Geometry: final body of the model. Coordinates: model frame, mm. A direction names the side the tool comes from. Give positions to 0.01 mm unless a question says otherwise; leave off trailing zeros. Write each loop counter-clockwise with the first axis right and the second up, starting at its lowest first coordinate (ties: lowest second). Pieces come first, ordered by that corner, then holes. Notation, with made-up numbers: (-30.75, -5.5) -> (-12.75, -5.5) arc R23 ccw to (-12.75, 13.5) -> close; hole circle Ø11 at (10, 25). An arc over 180 degrees is marked (long way). Answer as a JSON object with one key per item and string values. Group by question number.
(1) Contact query for flat-ended pins moving along their axis: pin 1 Ø6 at (x, y) = (8.5, 68) entering from +Z; pin 2 Ø7 at (x, z) = (-36.25, -33.1) entering from +Y. Output: stop coordinate, or through.
(2) Set-up query: faces 1 (the face through (44.424, 47.566, -5.07)), 2 (the face through (-0.79, 7.4, -35.99)), 3 (the face through (-39.2, 109.93, -30.39)). Return all of +Z, -Z, +X, -X, +Y, -Y with unobstructed straight access to the full face (end or side cutting, diameter ignored); none if empty.
(3) Section query A-A on y = 10. Output: boundary loops of the cut face in (x, z).
(4) Draft query along Y for faces 4 (the face through (35.73, 109.93, -29.13)), 5 (the face through (-38.076, 47.566, -5.07)), 6 (the face through (-1, 0, -41)). Return one class per face: +Y half, -Y half, draft (parallel to the pull), parting line (faces both ways), or undercut.
(5) Material intervals for probe 1 along Y at (x, z) = (-41, -5); probe 2 along X at (y, z) = (105.5, -34.5); probe 3 along X at (y, z) = (50, -5), sorted ascending.
(6) Section query B-B on x = 0. Output: boundary loops of the cut face in (y, z), plus the area to 4 significant figures.
from build123d import *

# Parameters (mm, degrees)
F2_DEPTH = 50
F5_D     = 8
F5_DEPTH = 10
F5_TIP   = 2.4034424761
F7_D     = 8
F7_DEPTH = 20
F7_TIP   = 2.4034424761
F8_DEPTH = 10


with BuildPart() as f2:
    # F1 (on Top) → F2 (new body)
    with BuildSketch(Plane.XY):
        Polygon((-50, 0), (0, 0), (50, 0), (50, 125), (-50, 125), align=None)
    extrude(amount=-F2_DEPTH)

    # F0 (on Top) → F3 (revolve, cut)
    with BuildSketch(Plane.XY):
        Polygon((-36, 0), (0, 0), (0, 125), (-32.5, 125), (-32.5, 35), (-36, 15), align=None)
    revolve(axis=Axis((0, 62.5, 0), (0, -1, 0)), mode=Mode.SUBTRACT)

    # F5
    with Locations(Plane.XY):
        with Locations((-41.25, 50), (41.25, 50)):
            Hole(F5_D / 2, depth=F5_DEPTH)
            with Locations((0, 0, -(F5_DEPTH + F5_TIP / 2))):  # 118° drill point
                Cone(0, F5_D / 2, F5_TIP, mode=Mode.SUBTRACT)

    # F7
    with Locations(Plane(origin=(0, 125, 0), x_dir=(-1, 0, 0), z_dir=(0, 1, 0))):
        with Locations((-36.2523114815, -33.0952695304), (36.2523114815, -33.0952695304)):
            Hole(F7_D / 2, depth=F7_DEPTH)
            with Locations((0, 0, -(F7_DEPTH + F7_TIP / 2))):  # 118° drill point
                Cone(0, F7_D / 2, F7_TIP, mode=Mode.SUBTRACT)

    # F8 (cut): a face of the model
    f8_faces = [f2.faces().sort_by_distance(p)[0] for p in [
        (41.25, 125, -1.1180339887),
    ]]
    extrude(f8_faces, amount=-F8_DEPTH, mode=Mode.SUBTRACT)


solid = f2.part
Answer list:
{
 "1": {"pin 1": "z = -30.4", "pin 2": "y = 104.7"},
 "2": {"face 1": "+Z", "face 2": "+Z, -Y", "face 3": "+Y"},
 "3": {"outline": "(-50, -50) -> (50, -50) -> (50, 0) -> (36, 0) arc R36 cw to (-36, 0) -> (-50, 0) -> close"},
 "4": {"face 4": "draft", "face 5": "undercut", "face 6": "-Y half"},
 "5": {"probe 1": "0 to 46.01, 53.99 to 115", "probe 2": "-50 to -40, -32.51 to 32.51, 40 to 50", "probe 3": "-50 to -45.25, -37.25 to -32.11, 32.11 to 37.25, 45.25 to 50"},
 "6": {"outline": "(0, -50) -> (115, -50) -> (115, -32.5) -> (35, -32.5) -> (15, -36) -> (0, -36) -> close", "area": "1,925 mm2"}
}
